Check sheet for the modelled part. Datum: model origin and axes. Units: mm. Coordinates: 2 decimals unless noted, no trailing zeros. Order: outer loops, then holes, each group sorted by start corner. A loop starts at its lowest first (then second) coordinate and runs counter-clockwise, first axis right, second up.
from build123d import *

# Parameters (mm, degrees)
SKETCH_1_R          = 11
SKETCH_1_R_2        = 5
EXTRUDE_1_DEPTH     = 12.5
SKETCH_2_R          = 1.6
CUT_EXTRUDE_1_DEPTH = 12.5


with BuildPart() as part:
    # ｽｹｯﾁ1 → ﾎﾞｽ - 押し出し1 (new, symmetric)
    with BuildSketch(Plane(origin=(0, 0, 0), x_dir=(1, 0, 0), z_dir=(0, 1, 0))):
        with Locations(Location((0, 0, 0), (0, 0, 270))):
            Circle(SKETCH_1_R)
        with Locations(Location((0, 0, 0), (0, 0, 270))):
            Circle(SKETCH_1_R_2, mode=Mode.SUBTRACT)
    extrude(amount=EXTRUDE_1_DEPTH, both=True)

    # ｽｹｯﾁ2 → ｶｯﾄ - 押し出し1 (cut, symmetric)
    with BuildSketch(Plane.XY):
        with Locations((0, 7.5)):
            Circle(SKETCH_2_R)
        with Locations((0, -7.5)):
            Circle(SKETCH_2_R)
    extrude(amount=CUT_EXTRUDE_1_DEPTH, both=True, mode=Mode.SUBTRACT)


solid = part.part
(1) Thickness scan on probe 1 along Y at (x, z) = (0, 6); probe 2 along X at (y, z) = (-4.5, 0); probe 3 along X at (y, z) = (-6.5, 8). Record the ranges inside material, lowest first.
Filled in:
probe 1: y = -12.5 to -9.1, -5.9 to 5.9, 9.1 to 12.5
probe 2: x = -11 to -5, 5 to 11
probe 3: x = -7.55 to -1.25, 1.25 to 7.55
(2) Cross-section at D-D (z = -8.25). Enter the section's corners in (x, y).
Filled in:
outline: (-7.28, -12.5) - (7.28, -12.5) - (7.28, 12.5) - (-7.28, 12.5) - close; hole circle Ø3.2 at (0, -7.5); hole circle Ø3.2 at (0, 7.5)
(3) Cross-section at B-B (x = 0). Enter the section's corners in (y, z), and give its area (3 significant figures).
Filled in:
outline: (-12.5, -11) - (-9.1, -11) - (-9.1, -5) - (-12.5, -5) - close; (-12.5, 5) - (-9.1, 5) - (-9.1, 11) - (-12.5, 11) - close; (-5.9, -11) - (5.9, -11) - (5.9, -5) - (-5.9, -5) - close; (-5.9, 5) - (5.9, 5) - (5.9, 11) - (-5.9, 11) - close; (9.1, -11) - (12.5, -11) - (12.5, -5) - (9.1, -5) - close; (9.1, 5) - (12.5, 5) - (12.5, 11) - (9.1, 11) - close
area: 223 mm2
(4) Go/stop test with flat-tipped pins: P1, Ø2, axis at y = -8, z = 7, coming from the +X side; P2, Ø6, axis at x = -6.5, y = -8, coming from the +Z side; P3, Ø3, axis at x = -0.5, z = 1.5, coming from the -Y side; P4, Ø6, axis at y = -8, z = -6.5, coming from the -X side. Record where each tip stops, or that it passes through.
Filled in:
P1: stops at x = 9.22
P2: stops at z = 10.43
P3: passes through
P4: stops at x = -10.43
(5) Release check for a two-part mould opening along Y. For faces 1 (the cylindrical face through (-0.35, -9.06, 7.91)), 2 (the flat face through (-5, -12.5, 2)), 3 (the flat face through (-5, 12.5, 2)) record: +Y half, -Y half, draft (parallel to the pull), parting line (faces both ways), or undercut.
Filled in:
face 1: undercut
face 2: -Y half
face 3: +Y half
(6) Cross-section at C-C (y = -7.5). Enter the section's corners in (x, z), and give its area (3 significant figures).
Filled in:
outline: (-1.6, -10.88) - (-1.6, -4.74) arc R5 cw to (-1.6, 4.74) - (-1.6, 10.88) arc R11 ccw to start; (1.6, -10.88) arc R11 ccw to (1.6, 10.88) - (1.6, 4.74) arc R5 cw to (1.6, -4.74) - close
area: 263 mm2
(7) Cross-section at A-A (z = 0). Enter the section's corners in (x, y), and give its area (3 significant figures).
Filled in:
outline: (-11, -12.5) - (-5, -12.5) - (-5, 12.5) - (-11, 12.5) - close; (5, -12.5) - (11, -12.5) - (11, 12.5) - (5, 12.5) - close
area: 300 mm2
